Answer from the drawing. Dimensions are ordinates in mm from the lowest x, y and z of the part. Give positions to 0.01 mm unless a question says otherwise; leave off trailing zeros. Write each loop counter-clockwise with the first axis right and the second up, starting at its lowest first coordinate (ties: lowest second). Pieces come first, ordered by that corner, then holes.
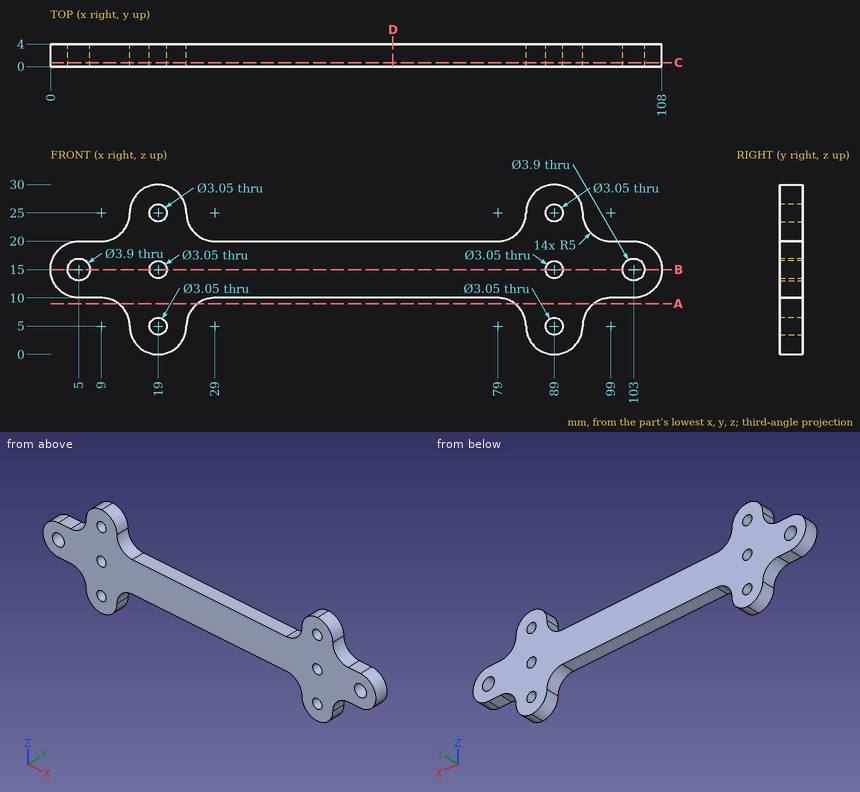
Item 1: Each of these flat-tipped pins is pushed along its axis until it touches: pin 1 Ø2.5 at (x, z) = (19, 5) entering from -Y; pin 2 Ø1.2 at (x, y) = (6.5, 3) entering from +Z; pin 3 Ø1 at (y, z) = (1.5, 8) entering from -X; pin 4 Ø1.5 at (y, z) = (1, 22.5) entering from -X. Where does it stop, or does it pass through?
Result set:
pin 1: passes through
pin 2: stops at z = 20
pin 3: stops at x = 12.57
pin 4: stops at x = 12.8
Item 2: Section B-B (z = 15) is taken. Write down the section's boundary in (x, y) (3 decimals), and give its area (3 significant figures).
Result set:
outline: (0, 0) - (3.05, 0) - (3.05, 4) - (0, 4) - close; (6.95, 0) - (17.475, 0) - (17.475, 4) - (6.95, 4) - close; (20.525, 0) - (87.475, 0) - (87.475, 4) - (20.525, 4) - close; (90.525, 0) - (101.05, 0) - (101.05, 4) - (90.525, 4) - close; (104.95, 0) - (108, 0) - (108, 4) - (104.95, 4) - close
area: 376 mm2
Item 3: Section D-D (x = 60.5) is taken. Write down the section's boundary in (y, z), and give its area (3 significant figures).
Result set:
outline: (0, 10) - (4, 10) - (4, 20) - (0, 20) - close
area: 40.0 mm2
Item 4: Find the intervals of material crossed by line 1 along X through (y, z) = (1.2, 15) (3 decimals); line 2 along X through (y, z) = (1, 25.25); line 3 along Z through (x, y) = (89, 1.7) (3 decimals), in increasing order.
Result set:
line 1: x = 0 to 3.05, 6.95 to 17.475, 20.525 to 87.475, 90.525 to 101.05, 104.95 to 108
line 2: x = 14.01 to 17.5, 20.5 to 23.99, 84.01 to 87.5, 90.5 to 93.99
line 3: z = 0 to 3.475, 6.525 to 13.475, 16.525 to 23.475, 26.525 to 30
Item 5: Section A-A (z = 9) is taken. Write down the section's boundary in (x, y).
Result set:
outline: (12, 0) - (26, 0) - (26, 4) - (12, 4) - close; (82, 0) - (96, 0) - (96, 4) - (82, 4) - close
Item 6: Section C-C (y = 0.7) is taken. Give the number of separate pieces and of enclosed holes in the cut face, and give its area (3 significant figures).
Result set:
separate pieces: 1
enclosed holes: 8
area: 1,390 mm2
